Build history of the part. All positions in model axes, mm. Give positions to 0.01 mm unless a question says otherwise; leave off trailing zeros. Loops run counter-clockwise (first coordinate to the right, second up) from the corner with the lowest first, then second, coordinate; pieces in that order, holes last. Notation, with made-up numbers: (16, 38.5) -> (32, 38.5) arc R25 cw to (32, 66.5) -> close; hole circle Ø9 at (34.5, -39.75). An arc over 180 degrees is marked (long way). One line per question, with ' | ' between items. Start each with the question number.
(1) Slice it at A-A, the plane z = 0. Write the cut outline in (x, y), then the cut area to 3 significant figures.
(2) Flat gauge pins, fed straight in: pin 1 Ø1.5 at (y, z) = (14, -45.5) entering from +X; pin 2 Ø10 at (y, z) = (56.5, 265.5) entering from -X; pin 3 Ø6 at (y, z) = (13, -163) entering from +X. Where does each tip first touch, or does it go through?
(3) Slice it at B-B, the plane y = 70. Give the number of separate pieces and of enclosed holes in the cut face, then the cut area to 3 significant figures.
(4) Drill centre lines: L1, parallel to X at y = 55, z = 0; L2, parallel to Z at x = 142, y = 66.5; L3, parallel to Z at x = 325.5, y = 69.5. Where is each one in solid material? Low to high. Write a range as from..to.
(5) Slice it at C-C, the plane y = 11. Write the cut outline in (x, z).
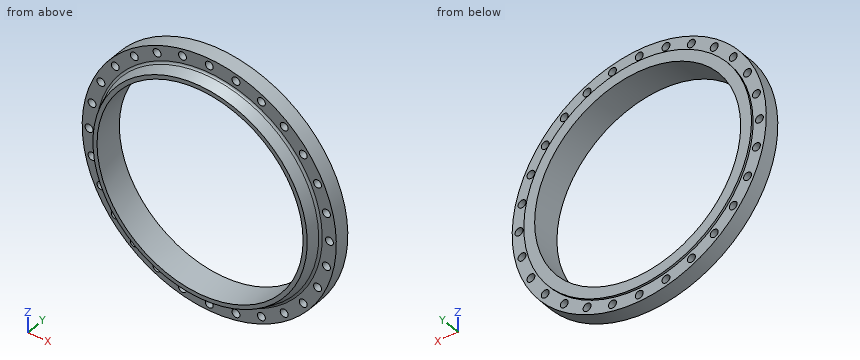
```python
from build123d import *

# Parameters (mm, degrees)
SKETCH_2_R          = 11.5
CUT_EXTRUDE_1_DEPTH = 530.189002153
SKETCH1_R           = 300
CUT_EXTRUDE1_DEPTH  = 529.606659058


with BuildPart() as part:
    # Sketch 1 → Revolve 1 (revolve)
    with BuildSketch(Plane.XY, mode=Mode.PRIVATE) as revolve_1_sk:
        with BuildLine():
            Line((-300, 0), (-300, 35))
            Line((-300, 35), (0, 35))
            Line((0, 35), (0, 75))
            Line((0, 75), (-300, 75))
            Line((-300, 75), (-300, 85))
            Line((-300, 85), (-331.5, 85))
            Line((-331.5, 85), (-331.5, 79))
            Line((-331.5, 79), (-370, 79))
            Line((-370, 79), (-370, 35))
            Line((-370, 35), (-329, 35))
            ThreePointArc((-329, 35), (-324.931332644, 33.696134298), (-322.378378378, 30.27027027))
            Line((-322.378378378, 30.27027027), (-312, 0))
            Line((-312, 0), (-300, 0))
        make_face()
    revolve(revolve_1_sk.sketch.rotate(Axis((0, 0, 0), (0, 1, 0)), 270), axis=Axis((0, 0, 0), (0, 1, 0)))

    # Sketch 2 → Cut-Extrude 1 (cut, through all)
    with BuildSketch(Plane(origin=(0, 79, 0), x_dir=(1, 0, 0), z_dir=(0, 1, 0))):
        with Locations(Location((0, 350, 0), (0, 0, 270))):
            Circle(SKETCH_2_R)
        with Locations(Location((77.882326885, 341.224769264, 0), (0, 0, 270))):
            Circle(SKETCH_2_R)
        with Locations(Location((151.859308691, 315.339103766, 0), (0, 0, 270))):
            Circle(SKETCH_2_R)
        with Locations(Location((218.221430651, 273.641018864, 0), (0, 0, 270))):
            Circle(SKETCH_2_R)
        with Locations(Location((273.641018864, 218.221430651, 0), (0, 0, 270))):
            Circle(SKETCH_2_R)
        with Locations(Location((315.339103766, 151.859308691, 0), (0, 0, 270))):
            Circle(SKETCH_2_R)
        with Locations(Location((341.224769264, 77.882326885, 0), (0, 0, 270))):
            Circle(SKETCH_2_R)
        with Locations(Location((350, 0, 0), (0, 0, 270))):
            Circle(SKETCH_2_R)
        with Locations(Location((341.224769264, -77.882326885, 0), (0, 0, 270))):
            Circle(SKETCH_2_R)
        with Locations(Location((315.339103766, -151.859308691, 0), (0, 0, 270))):
            Circle(SKETCH_2_R)
        with Locations(Location((273.641018864, -218.221430651, 0), (0, 0, 270))):
            Circle(SKETCH_2_R)
        with Locations(Location((218.221430651, -273.641018864, 0), (0, 0, 270))):
            Circle(SKETCH_2_R)
        with Locations(Location((151.859308691, -315.339103766, 0), (0, 0, 270))):
            Circle(SKETCH_2_R)
        with Locations(Location((77.882326885, -341.224769264, 0), (0, 0, 270))):
            Circle(SKETCH_2_R)
        with Locations(Location((0, -350, 0), (0, 0, 270))):
            Circle(SKETCH_2_R)
        with Locations(Location((-77.882326885, -341.224769264, 0), (0, 0, 270))):
            Circle(SKETCH_2_R)
        with Locations(Location((-151.859308691, -315.339103766, 0), (0, 0, 270))):
            Circle(SKETCH_2_R)
        with Locations(Location((-218.221430651, -273.641018864, 0), (0, 0, 270))):
            Circle(SKETCH_2_R)
        with Locations(Location((-273.641018864, -218.221430651, 0), (0, 0, 270))):
            Circle(SKETCH_2_R)
        with Locations(Location((-315.339103766, -151.859308691, 0), (0, 0, 270))):
            Circle(SKETCH_2_R)
        with Locations(Location((-341.224769264, -77.882326885, 0), (0, 0, 270))):
            Circle(SKETCH_2_R)
        with Locations(Location((-350, 0, 0), (0, 0, 270))):
            Circle(SKETCH_2_R)
        with Locations(Location((-341.224769264, 77.882326885, 0), (0, 0, 270))):
            Circle(SKETCH_2_R)
        with Locations(Location((-315.339103766, 151.859308691, 0), (0, 0, 270))):
            Circle(SKETCH_2_R)
        with Locations(Location((-273.641018864, 218.221430651, 0), (0, 0, 270))):
            Circle(SKETCH_2_R)
        with Locations(Location((-218.221430651, 273.641018864, 0), (0, 0, 270))):
            Circle(SKETCH_2_R)
        with Locations(Location((-151.859308691, 315.339103766, 0), (0, 0, 270))):
            Circle(SKETCH_2_R)
        with Locations(Location((-77.882326885, 341.224769264, 0), (0, 0, 270))):
            Circle(SKETCH_2_R)
    extrude(amount=-CUT_EXTRUDE_1_DEPTH, mode=Mode.SUBTRACT)

    # Sketch1 → Cut-Extrude1 (cut, through all)
    with BuildSketch(Plane(origin=(0, 75, 0), x_dir=(1, 0, 0), z_dir=(0, 1, 0))):
        with Locations(Location((0, 0, 0), (0, 0, 90))):
            Circle(SKETCH1_R)
    extrude(amount=-CUT_EXTRUDE1_DEPTH, mode=Mode.SUBTRACT)


solid = part.part
```
Final values:
1) outline: (-370, 35) -> (-361.5, 35) -> (-361.5, 79) -> (-370, 79) -> close; (-338.5, 35) -> (-329, 35) arc R7 cw to (-322.38, 30.27) -> (-312, 0) -> (-300, 0) -> (-300, 85) -> (-331.5, 85) -> (-331.5, 79) -> (-338.5, 79) -> close; (300, 0) -> (312, 0) -> (322.38, 30.27) arc R7 cw to (329, 35) -> (338.5, 35) -> (338.5, 79) -> (331.5, 79) -> (331.5, 85) -> (300, 85) -> close; (361.5, 35) -> (370, 35) -> (370, 79) -> (361.5, 79) -> close | area: 5,780 mm2
2) pin 1: x = 313.8 | pin 2: x = -262.75 | pin 3: x = 273.4
3) separate pieces: 1 | enclosed holes: 29 | area: 136,000 mm2
4) L1: -370..-361.5, -338.5..-300, 300..338.5, 361.5..370 | L2: -341.67..-321.26, -309.42..-264.27, 264.27..309.42, 321.26..341.67 | L3: -175.93..-157.25, -146.47..146.47, 157.25..175.93
5) outline: circle Ø631.54 at (0, 0); hole circle Ø600 at (0, 0)
